Can you work these out from the model? Positions are in its coordinate system, mm. A direction names the side the tool comes from. Give positions to 0.01 mm unless a question says otherwise; leave off trailing zeros. Loops run counter-clockwise (first coordinate to the right, second up) from the corner with the lowest first, then second, coordinate; pieces in that order, holes last. Notation, with made-up numbers: (33, -37) - (41, -37) arc R20 ccw to (41, -16) - close; hole circle Ø2 at (53, -38). An arc over 180 degrees is marked (long way). Answer in a Markdown table with one row per item.
Autodesk Inventor part; units mm, degrees
ref_plane "YZ Plane" through (0, 0, 0) normal (1, 0, 0) x (0, 1, 0)
ref_plane "XZ Plane" through (0, 0, 0) normal (0, 1, 0) x (-1, 0, 0)
ref_plane "XY Plane" through (0, 0, 0) normal (0, 0, 1) x (1, 0, 0)
sketch "Sketch1" plane through (0, 0, 0) normal (0, 1, 0) x (-1, 0, 0)
  line L0 (0, 0) -> (-304.8, 0)
  line L1 (-304.8, 0) -> (-304.8, -76.2)
  line L2 (-304.8, -76.2) -> (0, -76.2)
  line L3 (0, -76.2) -> (0, 0)
  line L4 (-152.4, -76.2) -> (-152.4, 0)
  line L5 (-304.8, -38.1) -> (0, -38.1)
  line L6 (-127, -50.8) -> (-177.8, -50.8)
  line L7 (-177.8, -50.8) -> (-177.8, -25.4)
  line L8 (-177.8, -25.4) -> (-127, -25.4)
  line L9 (-127, -25.4) -> (-127, -50.8)
  line L10 (-127, -50.8) -> (-177.8, -25.4) construction
  line L11 (-177.8, -50.8) -> (-127, -25.4) construction
  line L12 (-120.65, -57.15) -> (-184.15, -57.15) construction
  line L13 (-184.15, -57.15) -> (-184.15, -19.05) construction
  line L14 (-184.15, -19.05) -> (-120.65, -19.05) construction
  line L15 (-120.65, -19.05) -> (-120.65, -57.15) construction
  circle A0 centre (-120.65, -57.15) radius 1.5875
  circle A1 centre (-184.15, -57.15) radius 1.5875
  circle A2 centre (-120.65, -19.05) radius 1.5875
  circle A3 centre (-184.15, -19.05) radius 1.5875
  point P0 (-6.35, -69.85)
  point P1 (-152.4, -38.1)
  point P2 (-6.35, -69.85)
  point P3 (-298.45, -69.85)
  point P4 (-6.35, -6.35)
  point P5 (-298.45, -6.35)
  point P6 (-152.4, -6.35)
  dimension "d0" = 76.2
  dimension "d1" = 304.8
  dimension "d5" = 6.35
  dimension "d6" = 6.35
  dimension "d16" = 50.8
  dimension "d17" = 25.4
  dimension "d19" = 6.35
  dimension "d20" = 3.175
extrude "Extrusion1" add sketch "Sketch1" against normal blind 12.7 contours L3 L5 L9 L8 L4 L0 | L4 L8 L7 L5 L1 L0 | L3 L2 L4 L6 L9 L5 | L5 L7 L6 L4 L2 L1 | A0 | A1 | A2 | A3
hole "Mounting Hole" at (6.35, 0, -69.85) direction (0, -1, 0) diameter 3.2766 end through all countersink diameter 5.715 countersink angle 82
pattern_sketch "Mounting Holes" of "Mounting Hole" from (6.35, 0, -69.85) copies at (298.45, 0, -69.85) at (298.45, 0, -6.35) at (6.35, 0, -6.35) at (152.4, 0, -6.35)
sketch "Sketch2" plane through (0, 0, 0) normal (0, 1, 0) x (1, 0, 0)
  point P0 (120.65, 57.15)
  point P1 (120.65, 19.05)
  point P2 (184.15, 19.05)
  point P3 (184.15, 57.15)
hole "Jack Plate Mounting" at (120.65, 0, -57.15) direction (0, -1, 0) diameter 3.81 end through all
pattern_sketch "Jack Plate Mounting Holes" of "Jack Plate Mounting" from (120.65, 0, -57.15) copies at (120.65, 0, -19.05) at (184.15, 0, -19.05) at (184.15, 0, -57.15)
fillet "Fillet1" radius 6.35 4 edges at (127, -6.35, -50.8) (127, -6.35, -25.4) (177.8, -6.35, -25.4) (177.8, -6.35, -50.8)
properties material "MDF Medium Density Fiberboard"
Q1. Imagine slicing it at B-B, the plane x = 174. Write out the boundary of the cut face in (y, z).
Checked values:
| item | result |
|---|---|
| outline | (-12.7, -76.2) - (0, -76.2) - (0, -50.27) - (-12.7, -50.27) - close; (-12.7, -25.93) - (0, -25.93) - (0, 0) - (-12.7, 0) - close |
Q2. For pin 1 (3 mm diameter, centred on x = 6.35, z = -69.85, fed in from -Y); pin 2 (4 mm diameter, centred on x = 152.4, z = -6.35, fed in from +Y), each with a flat end and sliding along its axis, tell me the tip position at first contact or that it passes through.
Checked values:
| item | result |
|---|---|
| pin 1 | passes through |
| pin 2 | stops at y = -0.99 |
Q3. If we mould it in two halves opening along X, with no side actions, what happens to faces 1 (the face through (127, -6, -38)), 2 (the face through (155, -12.7, -54)), 3 (the face through (0, -6, -39))? For each: released by +X, released by -X, zero draft, split by the parting line, or undercut.
Checked values:
| item | result |
|---|---|
| face 1 | undercut |
| face 2 | zero draft |
| face 3 | released by -X |
Q4. If I drill on line 1 (Z direction, x = 184.15, y = -6.75) (3 decimals); line 2 (X direction, y = -9.5, z = -69.85); line 3 (X direction, y = -7.25, z = -19.05) (3 decimals), over which ranges is the centre line in solid material (lowest first)? Write a range as [from, to].
Checked values:
| item | result |
|---|---|
| line 1 | z = [-76.2, -59.055], [-55.245, -20.955], [-17.145, 0] |
| line 2 | x = [0, 4.71], [7.99, 296.81], [300.09, 304.8] |
| line 3 | x = [0, 118.745], [122.555, 182.245], [186.055, 304.8] |
Q5. Imagine slicing it at A-A, the plane y = -10. Count the separate pieces of the cut face and the enclosed holes in it, and give its area (3 significant figures).
Checked values:
| item | result |
|---|---|
| separate pieces | 1 |
| enclosed holes | 10 |
| area | 21,900 mm² |
Q6. On a 3-axis mill with a long thin cutter (end or side, diameter ignored), from which of +Z, -Z, +X, -X, +Y, -Y can I reach the whole of each face in a straight line? I mean faces 4 (the face through (155, -6, -76.2)), 5 (the face through (177.8, -6, -38)). Say none if no direction works.
Checked values:
| item | result |
|---|---|
| face 4 | -Z, +X, -X, +Y, -Y |
| face 5 | +Y, -Y |
